Read the model definition and answer for the solid it produces. Units are mm, in the model's axes. A direction names the side the tool comes from. Coordinates: 2 decimals unless noted, no trailing zeros. Loops run counter-clockwise (first coordinate to the right, second up) from the corner with the lowest first, then second, coordinate; pieces in that order, holes last. Notation, with made-up numbers: (65, 62.5) - (111, 62.5) arc R26 ccw to (111, 95.5) - close; hole circle Ø1 at (-10.5, 64). An arc over 180 degrees is marked (long way). Use CSV: the item, a comma, the result in double quotes.
Autodesk Inventor part; units mm, degrees
ref_plane "YZ Plane" through (0, 0, 0) normal (1, 0, 0) x (0, 1, 0)
ref_plane "XZ Plane" through (0, 0, 0) normal (0, 1, 0) x (-1, 0, 0)
ref_plane "XY Plane" through (0, 0, 0) normal (0, 0, 1) x (1, 0, 0)
sketch "Sketch1" plane through (0, 0, 0) normal (0, 1, 0) x (-1, 0, 0)
  arc A0 (-1.5, 9.2569) -> (1.5, 9.2569) centre (0, 4.75) ccw
  arc A1 (5.3889, -0.1) -> (4.5, 10.4344) centre (0, 4.75) ccw
  arc A2 (-4.5, 10.4344) -> (-5.3889, -0.1) centre (0, 4.75) ccw
  line L0 (-4.5, 10.4344) -> (-4.5, 17.9344)
  line L1 (4.5, 10.4344) -> (4.5, 17.9344)
  line L2 (-1.5, 9.2569) -> (-1.5, 17.9344)
  line L3 (1.5, 9.2569) -> (1.5, 17.9344)
  line L4 (4.5, 17.9344) -> (1.5, 17.9344)
  line L5 (-1.5, 17.9344) -> (-4.5, 17.9344)
  line L6 (5.3889, -0.1) -> (-5.3889, -0.1)
  point P0 (0, 0)
extrude "Extrusion1" add sketch "Sketch1" along normal blind 10
sketch "Sketch2" plane through (0, 0, 0) normal (0, 1, 0) x (-1, 0, 0)
  line L0 (-5.3889, -0.1) -> (5.3889, -0.1)
  line L1 (0, -0.1) -> (-10, -0.1)
  line L2 (0, -0.1) -> (10, -0.1)
  line L3 (-10, -0.1) -> (-10, -7.1)
  line L4 (-10, -7.1) -> (10, -7.1)
  line L5 (10, -7.1) -> (10, -0.1)
  point P0 (0, 0)
  dimension "d13" = 10
  dimension "d14" = 10
  dimension "d15" = 7
  dimension "d16" = 20
  dimension "d17" = 7
extrude "Extrusion2" add sketch "Sketch2" along normal blind 25 and the other way blind 15
sketch "Sketch3" plane through (0, 25, 0) normal (0, 1, 0) x (1, 0, 0)
  line L0 (-10, 0.1) -> (10, 0.1)
  line L1 (10, 7.1) -> (10, 0.1)
  circle A0 centre (7, 3.6) radius 1.5
  line L2 (-10, 7.1) -> (-10, 0.1)
  circle A1 centre (-7, 3.6) radius 1.5
  point P0 (0, 0)
  dimension "d24" = 3
  dimension "d27" = 3
hole "Hole1" at (-7, 25, -3.6) at (7, 25, -3.6) direction (0, -1, 0) diameter 3 end through all both
sketch "Sketch4" plane through (4.5, 0, 17.9344) normal (1, 0, 0) x (0, 0, -1)
  line L0 (0, 10) -> (8.6775, 10)
  circle A0 centre (3.75, 5) radius 1.5
  point P0 (17.9344, 0)
  point P1 (0, 0)
  point P2 (7.5, 0)
  dimension "d36" = 3
hole "Hole2" at (4.5, 5, 14.1844) direction (-1, 0, 0) diameter 3 end through all both
Q1. Find the intervals of material crossed by probe 1 along X at (y, z) = (13.5, -3.6); probe 2 along Z at (x, y) = (7, 14); probe 3 along Z at (x, y) = (-3.6, 5), in increasing order. Write a range as [from, to].
Reported:
probe 1,"x = [-10, -8.5], [-5.5, 5.5], [8.5, 10]"
probe 2,"z = [-7.1, -5.1], [-2.1, -0.1]"
probe 3,"z = [-7.1, 1.65], [7.85, 12.68], [15.68, 17.93]"
Q2. Given P1, Ø1, axis at y = 0.5, z = 4.5, coming from the -X side; P2, Ø4.5, axis at y = 5.5, z = 14, coming from the -X side; P3, Ø8, axis at x = 6.5, z = 4, coming from the +Y side, each flat-ended and moving along its own axis, determine where each tip first touches the part or whether it passes through.
Reported:
P1,"stops at x = -7.25"
P2,"stops at x = -4.5"
P3,"stops at y = 10"
Q3. The part is cut by section D-D on y = -1. Determine the outline of the cut face in (x, z).
Reported:
outline,"(-10, -7.1) - (10, -7.1) - (10, -0.1) - (-10, -0.1) - close; hole circle Ø3 at (-7, -3.6); hole circle Ø3 at (7, -3.6)"
Q4. A tool of negligible diameter and unlimited length cuts with its end or side. For faces 4 (the face through (-4.5, 5, 16)), 5 (the face through (1.5, 3.8, 12.6)), 6 (the face through (2, 10, 11)), from which of +Z, -Z, +X, -X, +Y, -Y can it reach the whole face along a straight path? Write none if from no direction.
Reported:
face 4,"+Z, -X, +Y, -Y"
face 5,"+Z, +Y, -Y"
face 6,"+Z, +X, -X, +Y"
Q5. The part is cut by section C-C on x = 0. Determine the outline of the cut face in (y, z).
Reported:
outline,"(-15, -7.1) - (25, -7.1) - (25, -0.1) - (10, -0.1) - (10, 0) - (0, 0) - (0, -0.1) - (-15, -0.1) - close"
Q6. The part is cut by section B-B on y = 4. Determine the outline of the cut face in (x, z).
Reported:
outline,"(-10, -7.1) - (10, -7.1) - (10, -0.1) - (5.39, -0.1) arc R7.25 ccw to (4.5, 10.43) - (4.5, 13.07) - (1.5, 13.07) - (1.5, 9.26) arc R4.75 cw (long way) to (-1.5, 9.26) - (-1.5, 13.07) - (-4.5, 13.07) - (-4.5, 10.43) arc R7.25 ccw to (-5.39, -0.1) - (-10, -0.1) - close; (-4.5, 15.3) - (-1.5, 15.3) - (-1.5, 17.93) - (-4.5, 17.93) - close; (1.5, 15.3) - (4.5, 15.3) - (4.5, 17.93) - (1.5, 17.93) - close; hole circle Ø3 at (-7, -3.6); hole circle Ø3 at (7, -3.6)"
Q7. For a pull along Y with two mould halves and no side action, classify faces 1 (the face through (2, 0, 11)), 2 (the face through (-3.021, 4.549, 12.754)), 3 (the face through (-1.5, 3.8, 12.6)) as +Y half, -Y half, draft (parallel to the pull), parting line (faces both ways), or undercut.
Reported:
face 1,"-Y half"
face 2,"undercut"
face 3,"draft"
Q8. The part is cut by section A-A on z = -3.6. Determine the outline of the cut face in (x, y), and give its area (3 significant figures).
Reported:
outline,"(-10, -15) - (-8.5, -15) - (-8.5, 25) - (-10, 25) - close; (-5.5, -15) - (5.5, -15) - (5.5, 25) - (-5.5, 25) - close; (8.5, -15) - (10, -15) - (10, 25) - (8.5, 25) - close"
area,"560 mm²"
